Read the model definition and answer for the solid it produces. Units are mm, in the model's axes. Face numbers are marked on the shaded views. A direction names the side the tool comes from. Coordinates: 2 decimals unless noted, no trailing zeros. Loops run counter-clockwise (first coordinate to the right, second up) from the corner with the lowest first, then second, coordinate; pieces in that order, holes last. Notation, with made-up numbers: M -21,69.5 L -4,69.5 A23 ccw -4,77.5 Z; hole C 87.25,0.5 d5. An arc over 180 degrees is marked long. Put each result on its own line as item: value.
from build123d import *

# Parameters (mm, degrees)
F0_R     = 6.35
F0_W     = 25.4
F0_H     = 38.1
F1_DEPTH = 12.7
F2_DEPTH = 25.4


with BuildPart() as f1:
    # F0 (on Front) → F1 (new body)
    with BuildSketch(Plane.XZ):
        with BuildLine():
            ThreePointArc((-1.41771, -25.360404), (17.452079, -18.454943), (25.4, 0))
            ThreePointArc((25.4, 0), (17.452079, 18.454943), (-1.41771, 25.360404))
            ThreePointArc((-1.41771, 25.360404), (-25.4, 0), (-1.41771, -25.360404))
        make_face()
        Circle(F0_R, mode=Mode.SUBTRACT)
        with BuildLine():
            ThreePointArc((-1.41771, -25.360404), (-25.4, 0), (-1.41771, 25.360404))
            Line((-1.41771, 25.360404), (-14.828552, 24.610704))
            ThreePointArc((-14.828552, 24.610704), (-28.732781, 0), (-14.828552, -24.610704))
            Line((-14.828552, -24.610704), (-1.41771, -25.360404))
        make_face()
        with BuildLine():
            ThreePointArc((-14.828552, -24.610704), (-28.732781, 0), (-14.828552, 24.610704))
            Line((-14.828552, 24.610704), (-114.3, 19.05))
            Line((-114.3, 19.05), (-114.3, -19.05))
            Line((-114.3, -19.05), (-14.828552, -24.610704))
        make_face()
        with Locations((-127, 0)):
            Rectangle(F0_W, F0_H)
        with Locations((-127, -8.89)):
            Circle(F0_R, mode=Mode.SUBTRACT)
        with Locations((-127, 8.89)):
            Circle(F0_R, mode=Mode.SUBTRACT)
    extrude(amount=F1_DEPTH)

    # F0 (on Front) → F2 (join)
    with BuildSketch(Plane.XZ):
        with BuildLine():
            ThreePointArc((-14.828552, -24.610704), (-28.732781, 0), (-14.828552, 24.610704))
            Line((-14.828552, 24.610704), (-114.3, 19.05))
            Line((-114.3, 19.05), (-114.3, -19.05))
            Line((-114.3, -19.05), (-14.828552, -24.610704))
        make_face()
        with Locations((-127, 0)):
            Rectangle(F0_W, F0_H)
        with Locations((-127, -8.89)):
            Circle(F0_R, mode=Mode.SUBTRACT)
        with Locations((-127, 8.89)):
            Circle(F0_R, mode=Mode.SUBTRACT)
    extrude(amount=F2_DEPTH)


solid = f1.part
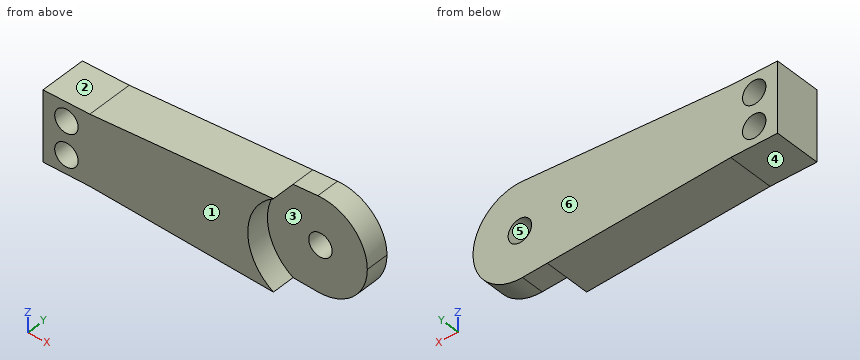
1) Find section C-C, the plane x = 0. Write down the section's boundary in (y, z).
Answer list:
outline: M -12.7,-25.4 L 0,-25.4 L 0,-6.35 L -12.7,-6.35 Z; M -12.7,6.35 L 0,6.35 L 0,25.4 L -12.7,25.4 Z
2) Which of the six approach directions +Z, -Z, +X, -X, +Y, -Y give full straight-line access (tool end or side, diameter ignored) to the marked faces 1, 2 and 3?
Answer list:
face 1: +Z, -Z, +X, -X, -Y
face 2: +Z, -X, +Y, -Y
face 3: +X, -Y
3) Given pin 1 Ø1 at (y, z) = (-22, -16.5) entering from +X; pin 2 Ø6 at (x, y) = (-103, -19) entering from -Z; pin 3 Ø1 at (y, z) = (-7, 6.5) entering from +X; pin 4 Ø14.5 at (x, z) = (-127, 8.89) entering from +Y, each flat-ended and moving along its own axis, determine where each tip first touches the part or whether it passes through.
Answer list:
pin 1: stops at x = -23.16
pin 2: stops at z = -19.85
pin 3: stops at x = 24.68
pin 4: stops at y = 0
4) Find section D-D, the plane y = -8.75. Write down the section's boundary in (x, z).
Answer list:
outline: M -139.7,-19.05 L -114.3,-19.05 L -1.42,-25.36 A25.4 ccw 25.4,0 A25.4 ccw -1.42,25.36 L -114.3,19.05 L -139.7,19.05 Z; hole C -127,-8.89 d12.7; hole C -127,8.89 d12.7; hole C 0,0 d12.7
5) Determine the mould class of the marked faces 4, 5 and 6 for opening direction Z: released by +Z, released by -Z, zero draft, split by the parting line, or undercut.
Answer list:
face 4: released by -Z
face 5: undercut
face 6: zero draft
6) Find section A-A, the plane x = -127. Write down the section's boundary in (y, z).
Answer list:
outline: M -25.4,-19.05 L 0,-19.05 L 0,-15.24 L -25.4,-15.24 Z; M -25.4,-2.54 L 0,-2.54 L 0,2.54 L -25.4,2.54 Z; M -25.4,15.24 L 0,15.24 L 0,19.05 L -25.4,19.05 Z
7) Find section B-B, the plane y = -23.25. Write down the section's boundary in (x, z).
Answer list:
outline: M -139.7,-19.05 L -114.3,-19.05 L -14.83,-24.61 A28.73 cw -14.83,24.61 L -114.3,19.05 L -139.7,19.05 Z; hole C -127,-8.89 d12.7; hole C -127,8.89 d12.7
8) Straight lines are drawn through the part: line 1 (Z direction, x = -127, y = -13.5); line 2 (Z direction, x = -126.5, y = -18.5); line 3 (Z direction, x = 0, y = -7.5). For each, find the intervals that lie inside material, in ascending order. Write a range as [from, to].
Answer list:
line 1: z = [-19.05, -15.24], [-2.54, 2.54], [15.24, 19.05]
line 2: z = [-19.05, -15.22], [-2.56, 2.56], [15.22, 19.05]
line 3: z = [-25.4, -6.35], [6.35, 25.4]
